from build123d import *

# Parameters (mm, degrees)
SKETCH2_R           = 3
SKETCH2_R_2         = 2
SKETCH2_R_3         = 12
BOSS_EXTRUDE1_DEPTH = 10


with BuildPart() as part:
    # Sketch2 → Boss-Extrude1 (new body)
    with BuildSketch(Plane.XY):
        with BuildLine():
            Line((16.086311, 54.546287057), (-73.913689, 54.546287057))
            ThreePointArc((-73.913689, 54.546287057), (-79.758605223, 49.901629949), (-76.554310886, 43.158605175))
            ThreePointArc((-76.554310886, 43.158605175), (-74.512035752, 41.314376729), (-73.754829124, 38.668870274))
            Line((-73.754829124, 38.668870274), (-73.754829124, 8.833412185))
            ThreePointArc((-73.754829124, 8.833412185), (-74.03645611, 7.179037348), (-74.849611564, 5.711029151))
            Line((-74.849611564, 5.711029151), (-94.607657852, -9.725648422))
            ThreePointArc((-94.607657852, -9.725648422), (-95.736830164, -18.022649664), (-87.472230382, -19.368625209))
            Line((-87.472230382, -19.368625209), (-9.642261307, 35.128505836))
            ThreePointArc((-9.642261307, 35.128505836), (-8.887470434, 35.56428455), (-8.06847435, 35.862374746))
            Line((-8.06847435, 35.862374746), (17.63922527, 42.750732099))
            ThreePointArc((17.63922527, 42.750732099), (22.034980168, 49.32944421), (16.086311, 54.546287057))
        make_face()
        with Locations((16.086311, 48.546287057)):
            Circle(SKETCH2_R, mode=Mode.SUBTRACT)
        with Locations((1.086311, 48.546287057)):
            Circle(SKETCH2_R_2, mode=Mode.SUBTRACT)
        with Locations((-13.913689, 48.546287057)):
            Circle(SKETCH2_R_2, mode=Mode.SUBTRACT)
        with Locations((-73.913689, 48.546287057)):
            Circle(SKETCH2_R, mode=Mode.SUBTRACT)
        with Locations((-90.913689, -14.453712943)):
            Circle(SKETCH2_R, mode=Mode.SUBTRACT)
        with Locations((-53.913689, 29.546287057)):
            Circle(SKETCH2_R_3, mode=Mode.SUBTRACT)
    extrude(amount=BOSS_EXTRUDE1_DEPTH)


solid = part.part
Geometry check sheet. Reference: the model listing, model coordinates, mm. A direction names the side the tool comes from. Coordinates: 2 decimals unless noted, no trailing zeros. Write each loop counter-clockwise with the first axis right and the second up, starting at its lowest first coordinate (ties: lowest second). Pieces come first, ordered by that corner, then holes. Notation, with made-up numbers: (39.25, 33.5) -> (54.25, 33.5) arc R31 cw to (54.25, 67.5) -> close; hole circle Ø6 at (58.25, 25). An arc over 180 degrees is marked (long way). One line per question, with ' | ' between items.
1. Cross-section at A-A on y = 33.5. Record the cut outline in (x, z), and give its area (3 significant figures).
Answers:
outline: (-73.75, 0) -> (-65.24, 0) -> (-65.24, 10) -> (-73.75, 10) -> close; (-42.58, 0) -> (-11.97, 0) -> (-11.97, 10) -> (-42.58, 10) -> close | area: 391 mm²
2. Set-up check for faces 1 (the cylindrical face through (-74.03, 7.2, 4.93)), 2 (the flat face through (-49.1, 7.5, 4.9)): record each of +Z, -Z, +X, -X, +Y, -Y from which the full face is reachable in a straight line by a thin tool's end or side.
Answers:
face 1: +Z, -Z, -X | face 2: +Z, -Z, +X, -Y
3. Thickness scan on probe 1 along X at (y, z) = (49.5, 4.75); probe 2 along Y at (x, z) = (-74.5, 7.75); probe 3 along Y at (x, z) = (-54, 5). Record the ranges inside material, lowest first. Write a range as from..to.
Answers:
probe 1: x = -79.84..-76.76, -71.07..-15.67, -12.16..-0.67, 2.84..13.24, 18.93..22.01 | probe 2: y = -10.29..6.21, 41.29..45.6, 51.49..54.52 | probe 3: y = 4.07..17.55, 41.55..54.55
4. Cross-section at B-B on x = -72.5. Record the cut outline in (y, z), and give its area (3 significant figures).
Answers:
outline: (-8.88, 0) -> (45.9, 0) -> (45.9, 10) -> (-8.88, 10) -> close; (51.19, 0) -> (54.55, 0) -> (54.55, 10) -> (51.19, 10) -> close | area: 581 mm²
5. Cross-section at D-D on y = -7. Record the cut outline in (x, z).
Answers:
outline: (-91.12, 0) -> (-69.81, 0) -> (-69.81, 10) -> (-91.12, 10) -> close
6. Draft check along X on faces 3 (the cylindrical face through (-79.732, 50.011, 4.93)), 4 (the cylindrical face through (22.05, 49.21, 4.93)), 5 (the cylindrical face through (15.7, 51.52, 4.93)). Enter one of: +X half, -X half, draft (parallel to the pull), parting line (faces both ways), or undercut.
Answers:
face 3: -X half | face 4: +X half | face 5: undercut
7. Cross-section at C-C on z = 4. Record the cut outline in (x, y), and give its area (3 significant figures).
Answers:
outline: (-94.61, -9.73) arc R6 ccw to (-87.47, -19.37) -> (-9.64, 35.13) arc R5 cw to (-8.07, 35.86) -> (17.64, 42.75) arc R6 ccw to (16.09, 54.55) -> (-73.91, 54.55) arc R6 ccw to (-76.55, 43.16) arc R5 cw to (-73.75, 38.67) -> (-73.75, 8.83) arc R5 cw to (-74.85, 5.71) -> close; hole circle Ø6 at (-90.91, -14.45); hole circle Ø6 at (-73.91, 48.55); hole circle Ø24 at (-53.91, 29.55); hole circle Ø4 at (-13.91, 48.55); hole circle Ø4 at (1.09, 48.55); hole circle Ø6 at (16.09, 48.55) | area: 2,970 mm²
8. Depth check by flat-ended pin: pin 1 Ø4 at (x, z) = (-74.5, 9) entering from -Y; pin 2 Ø21.5 at (x, y) = (-53.91, 29.55) entering from +Z; pin 3 Ø1.5 at (y, z) = (4.5, 3.5) entering from +X; pin 4 Ø2 at (y, z) = (21.5, 4.5) entering from -X. Enter the tip coordinate at first touch or a pass-through.
Answers:
pin 1: stops at y = -11.69 | pin 2: passes through | pin 3: stops at x = -52.31 | pin 4: stops at x = -73.75
